from build123d import *

# Parameters (mm, degrees)
SKETCH1_W           = 1524
SKETCH1_H           = 914.4
BOSS_EXTRUDE1_DEPTH = 31.75
BOSS_EXTRUDE2_DEPTH = 679.45


with BuildPart() as part:
    # Sketch1 → Boss-Extrude1 (new body)
    with BuildSketch(Plane(origin=(0, 0, 0), x_dir=(1, 0, 0), z_dir=(0, 1, 0))):
        Rectangle(SKETCH1_W, SKETCH1_H)
    extrude(amount=-BOSS_EXTRUDE1_DEPTH)

    # Sketch2 → Boss-Extrude2 (add)
    with BuildSketch(Plane.XZ.offset(31.75)):
        with BuildLine():
            Line((-698.5, -342.9), (-698.5, -381))
            ThreePointArc((-698.5, -381), (-685.8, -393.7), (-673.1, -381))
            Line((-673.1, -381), (-673.1, -342.9))
            ThreePointArc((-673.1, -342.9), (-685.8, -330.2), (-698.5, -342.9))
        make_face()
        with BuildLine():
            Line((-698.5, 381), (-698.5, 342.9))
            ThreePointArc((-698.5, 342.9), (-685.8, 330.2), (-673.1, 342.9))
            Line((-673.1, 342.9), (-673.1, 381))
            ThreePointArc((-673.1, 381), (-685.8, 393.7), (-698.5, 381))
        make_face()
        with BuildLine():
            Line((673.1, 381), (673.1, 342.9))
            ThreePointArc((673.1, 342.9), (685.8, 330.2), (698.5, 342.9))
            Line((698.5, 342.9), (698.5, 381))
            ThreePointArc((698.5, 381), (685.8, 393.7), (673.1, 381))
        make_face()
        with BuildLine():
            Line((673.1, -342.9), (673.1, -381))
            ThreePointArc((673.1, -381), (685.8, -393.7), (698.5, -381))
            Line((698.5, -381), (698.5, -342.9))
            ThreePointArc((698.5, -342.9), (685.8, -330.2), (673.1, -342.9))
        make_face()
    extrude(amount=BOSS_EXTRUDE2_DEPTH)


solid = part.part
Model file for the job. Use its own axes, mm. A direction names the side the tool comes from. Give positions to 0.01 mm unless a question says otherwise; leave off trailing zeros. Order: outer loops, then holes, each group sorted by start corner. A loop starts at its lowest first (then second) coordinate and runs counter-clockwise, first axis right, second up. Notation, with made-up numbers: (71.25, 65) -> (129.25, 65) arc R24 ccw to (129.25, 80) -> close; hole circle Ø6 at (13, -5). An arc over 180 degrees is marked (long way). Use CSV: the item, a comma, the result in double quotes.
1. Drill centre lines: line 1 along X through (y, z) = (-470, 384); line 2 along Y through (x, z) = (-663.5, -233); line 3 along X through (y, z) = (-84.5, -337). Where is each one in solid material? Low to high. Write a range as from..to.
Outcome:
line 1,"-698.14..-673.46, 673.46..698.14"
line 2,"-31.75..0"
line 3,"-697.05..-674.55, 674.55..697.05"
2. Drop flat-ended pins along their axis: pin 1 (5 mm diameter, centred on x = -62.5, z = 55, fed in from -Y); pin 2 (19 mm diameter, centred on y = -472.5, z = -354, fed in from +X); pin 3 (19 mm diameter, centred on y = -435, z = 369.5, fed in from -X). Give the stop position or say it passes through.
Outcome:
pin 1,"y = -31.75"
pin 2,"x = 698.5"
pin 3,"x = -698.5"
3. Band-saw the part on C-C, the plane x = -604. Give the cut face in (y, z), then the cut area to 3 significant figures.
Outcome:
outline,"(-31.75, -457.2) -> (0, -457.2) -> (0, 457.2) -> (-31.75, 457.2) -> close"
area,"29,000 mm²"
4. Band-saw the part on B-B, the plane z = 191. Give the cut face in (x, y).
Outcome:
outline,"(-762, -31.75) -> (762, -31.75) -> (762, 0) -> (-762, 0) -> close"
5. Mould opens along X. For faces 6 (the flat face through (698.5, -367, 362)), 7 (the flat face through (-673.1, -367, -362)), 8 (the flat face through (-11, 0, -6)) say: +X half, -X half, draft (parallel to the pull), parting line (faces both ways), or undercut.
Outcome:
face 6,"+X half"
face 7,"undercut"
face 8,"draft"
6. Band-saw the part on A-A, the plane y = -625. Give the cut face in (x, z).
Outcome:
outline,"(-698.5, -381) arc R12.7 ccw to (-673.1, -381) -> (-673.1, -342.9) arc R12.7 ccw to (-698.5, -342.9) -> close; (-698.5, 342.9) arc R12.7 ccw to (-673.1, 342.9) -> (-673.1, 381) arc R12.7 ccw to (-698.5, 381) -> close; (673.1, -381) arc R12.7 ccw to (698.5, -381) -> (698.5, -342.9) arc R12.7 ccw to (673.1, -342.9) -> close; (673.1, 342.9) arc R12.7 ccw to (698.5, 342.9) -> (698.5, 381) arc R12.7 ccw to (673.1, 381) -> close"
7. 3-axis set-ups, long thin cutter, end or side, ignore diameter. For faces 1 (the flat face through (673.1, -367, -362)), 2 (the flat face through (698.5, -367, -362)), 3 (the flat face through (762, -16, 6)), 4 (the flat face through (-698.5, -367, 362)), 5 (the flat face through (-11, -16, 457.2)): which of +Z, -Z, +X, -X, +Y, -Y reach the whole face in a straight line?
Outcome:
face 1,"+Z, -Z, -Y"
face 2,"+Z, -Z, +X, -Y"
face 3,"+Z, -Z, +X, +Y, -Y"
face 4,"+Z, -Z, -X, -Y"
face 5,"+Z, +X, -X, +Y, -Y"
